```python
from build123d import *

# Parameters (mm, degrees)
SKETCH_1_R      = 1.5
EXTRUDE_1_DEPTH = 3
FILLET_1_R      = 1


with BuildPart() as part:
    # 草图1 → 凸台-拉伸1 (new body)
    with BuildSketch(Plane.XY):
        with BuildLine():
            ThreePointArc((-38.025, -15), (-37.171446609, -15.353553391), (-37.525, -14.5))
            Line((-37.525, -14.5), (-37.525, 6.5))
            ThreePointArc((-37.525, 6.5), (-37.171446609, 7.353553391), (-38.025, 7))
            Line((-38.025, 7), (-43.525, 7))
            Line((-43.525, 7), (-43.525, 19))
            Line((-43.525, 19), (-38.025, 19))
            ThreePointArc((-38.025, 19), (-37.171446609, 18.646446609), (-37.525, 19.5))
            Line((-37.525, 19.5), (-37.525, 39))
            Line((-37.525, 39), (37.525, 39))
            Line((37.525, 39), (37.525, 19.5))
            ThreePointArc((37.525, 19.5), (37.171446609, 18.646446609), (38.025, 19))
            Line((38.025, 19), (43.525, 19))
            Line((43.525, 19), (43.525, 7))
            Line((43.525, 7), (38.025, 7))
            ThreePointArc((38.025, 7), (37.171446609, 7.353553391), (37.525, 6.5))
            Line((37.525, 6.5), (37.525, -14.5))
            ThreePointArc((37.525, -14.5), (37.171446609, -15.353553391), (38.025, -15))
            Line((38.025, -15), (43.525, -15))
            Line((43.525, -15), (43.525, -27))
            Line((43.525, -27), (37.525, -27))
            Line((37.525, -27), (-37.525, -27))
            Line((-37.525, -27), (-43.525, -27))
            Line((-43.525, -27), (-43.525, -15))
            Line((-43.525, -15), (-38.025, -15))
        make_face()
        with Locations((34.525, -5)):
            Circle(SKETCH_1_R, mode=Mode.SUBTRACT)
        with Locations((34.525, 33)):
            Circle(SKETCH_1_R, mode=Mode.SUBTRACT)
        with Locations((-34.525, -15)):
            Circle(SKETCH_1_R, mode=Mode.SUBTRACT)
        with Locations((-34.525, -5)):
            Circle(SKETCH_1_R, mode=Mode.SUBTRACT)
        with Locations((-34.525, 13)):
            Circle(SKETCH_1_R, mode=Mode.SUBTRACT)
        with Locations((-34.525, 33)):
            Circle(SKETCH_1_R, mode=Mode.SUBTRACT)
        with Locations((34.525, 13)):
            Circle(SKETCH_1_R, mode=Mode.SUBTRACT)
        with Locations((34.525, -15)):
            Circle(SKETCH_1_R, mode=Mode.SUBTRACT)
    extrude(amount=EXTRUDE_1_DEPTH)

    # 圆角1
    fillet_1_edges = [part.edges().sort_by_distance(p)[0] for p in [
        (-37.525, -14.5, 1.5),
        (-37.525, 6.5, 1.5),
        (-38.025, 7, 1.5),
        (-43.525, 7, 1.5),
        (-43.525, 19, 1.5),
        (-38.025, 19, 1.5),
        (-37.525, 19.5, 1.5),
        (-37.525, 39, 1.5),
        (37.525, 39, 1.5),
        (37.525, 19.5, 1.5),
        (38.025, 19, 1.5),
        (43.525, 19, 1.5),
        (43.525, 7, 1.5),
        (38.025, 7, 1.5),
        (37.525, 6.5, 1.5),
        (37.525, -14.5, 1.5),
        (38.025, -15, 1.5),
        (43.525, -15, 1.5),
        (43.525, -27, 1.5),
        (-43.525, -27, 1.5),
        (-43.525, -15, 1.5),
        (-38.025, -15, 1.5),
    ]]
    fillet(fillet_1_edges, radius=FILLET_1_R)


solid = part.part
```
Geometry check sheet. Reference: the model listing, model coordinates, mm. A direction names the side the tool comes from. Coordinates: 2 decimals unless noted, no trailing zeros. Order: outer loops, then holes, each group sorted by start corner. A loop starts at its lowest first (then second) coordinate and runs counter-clockwise, first axis right, second up. Notation, with made-up numbers: M 22,61.25 L 79,61.25 A11 ccw 79,80.25 Z; hole C 62.25,55.25 d6. An arc over 180 degrees is marked long. One line per question, with ' | ' between items. Start each with the question number.
Item 1: Gauge pin test, flat ends, axial feed: pin 1 (0.9 mm diameter, centred on x = 41, z = 1.5, fed in from +Y); pin 2 (1.5 mm diameter, centred on y = -1, z = 2, fed in from +X) (3 decimals); pin 3 (0.9 mm diameter, centred on y = -8.5, z = 2, fed in from -X) (3 decimals). Record the tip position at first contact, or that the pin passes through.
Item 2: Set-up check for faces 4 (the flat face through (41, 19, 1)), 5 (the flat face through (-37.525, -4, 1)), 6 (the flat face through (41, -15, 1)), 7 (the flat face through (1, 6, 0)), 8 (the flat face through (-43.525, -21, 1)): record each of +Z, -Z, +X, -X, +Y, -Y from which the full face is reachable in a straight line by a thin tool's end or side.
Item 3: Draft check along X on faces 1 (the flat face through (43.525, 13, 1)), 2 (the flat face through (1, -27, 1)), 3 (the cylindrical face through (-36.024, 13.066, 1.479)). Enter one of: pulls with the +X half, pulls with the -X half, needs draft (parallel to the pull), parting line crosses it, or undercut.
Item 4: Cross-section at C-C on z = 1.55. State how many separate pieces and enclosed holes the cut face has, then the cut area to 3 significant figures.
Item 5: Material ranges on L1, parallel to X at y = 5, z = 1 (3 decimals); L2, parallel to Y at x = -38, z = 2, recorded low to high. Write a range as [from, to].
Item 6: Cross-section at B-B on y = 33. Enter the section's corners in (x, z) (3 decimals).
Item 7: Cross-section at D-D on y = 4. Enter the section's corners in (x, z) (3 decimals).
Item 8: Cross-section at A-A on y = 13. Enter the section's corners in (x, z) (3 decimals).
Findings:
1) pin 1: stops at y = 19 | pin 2: stops at x = 37.525 | pin 3: stops at x = -37.525
2) face 4: +Z, -Z, +X, +Y | face 5: +Z, -Z, -X | face 6: +Z, -Z, +X | face 7: -Z, +X, -X, +Y, -Y | face 8: +Z, -Z, -X, +Y, -Y
3) face 1: pulls with the +X half | face 2: needs draft | face 3: undercut
4) separate pieces: 1 | enclosed holes: 8 | area: 5,180 mm²
5) L1: x = [-37.525, 37.525] | L2: y = [-27, -15.23], [7.23, 18.77]
6) outline: M -37.525,0 L -36.025,0 L -36.025,3 L -37.525,3 Z; M -33.025,0 L 33.025,0 L 33.025,3 L -33.025,3 Z; M 36.025,0 L 37.525,0 L 37.525,3 L 36.025,3 Z
7) outline: M -37.525,0 L 37.525,0 L 37.525,3 L -37.525,3 Z
8) outline: M -43.525,0 L -36.025,0 L -36.025,3 L -43.525,3 Z; M -33.025,0 L 33.025,0 L 33.025,3 L -33.025,3 Z; M 36.025,0 L 43.525,0 L 43.525,3 L 36.025,3 Z
